from build123d import *

# Parameters (mm, degrees)
F0_R           = 4
F1_DEPTH       = 10
F3_D           = 10
F3_CSINK_D     = 12
F3_CSINK_ANGLE = 90
F4_D           = 10
F4_CSINK_D     = 12
F4_CSINK_ANGLE = 90
F6_D           = 5


with BuildPart() as f1:
    # F0 (on Front) → F1 (new body)
    with BuildSketch(Plane.XZ):
        Polygon((0, 0), (-275, 0), (-275, -150), (275, -150), (275, 0), (50, 0), align=None)
        with Locations((-49.989153, -111.041441)):
            Circle(F0_R, mode=Mode.SUBTRACT)
        with Locations((49.989153, -111.041441)):
            Circle(F0_R, mode=Mode.SUBTRACT)
        with Locations((-49.989153, -41.041441)):
            Circle(F0_R, mode=Mode.SUBTRACT)
        with Locations((49.989153, -41.041441)):
            Circle(F0_R, mode=Mode.SUBTRACT)
    extrude(amount=F1_DEPTH)

    # F3 (through all)
    with Locations(Plane.XZ.offset(10)):
        with Locations((-132.18379, -88.733308)):
            CounterSinkHole(F3_D / 2, F3_CSINK_D / 2, counter_sink_angle=F3_CSINK_ANGLE)

    # F4 (through all)
    with Locations(Plane.XZ.offset(10)):
        with Locations((-164.520353, -73.822677)):
            CounterSinkHole(F4_D / 2, F4_CSINK_D / 2, counter_sink_angle=F4_CSINK_ANGLE)

    # F6 (through all)
    with Locations(Plane.XZ.offset(10)):
        with Locations((133.962631, -73.108293)):
            Hole(F6_D / 2)


solid = f1.part
Geometry: final body of the model. Coordinates: model frame, mm. Give positions to 0.01 mm unless a question says otherwise; leave off trailing zeros. Answer as a JSON object with one key per item and string values.
1. Contact query for a flat-ended pin moving along its axis: pin 1 (8 mm diameter, centred on x = -164.52, z = -73.82, fed in from -Y). Output: stop coordinate, or through.
Ans:
{"pin 1": "passes through"}
2. Mould query, pull axis X, two halves, no side actions, for faces 1 (the cylindrical face through (-127.19, -4.44, -88.51)), 2 (the flat face through (-4, -10, -74)), 3 (the flat face through (-275, -5, -74)). Classes: pulls with the +X half, pulls with the -X half, needs draft (parallel to the pull), parting line crosses it, or undercut.
Ans:
{"face 1": "undercut", "face 2": "needs draft", "face 3": "pulls with the -X half"}
3. Ray query, probe 1 along Z at (x, y) = (-166.5, -4.5); probe 2 along Z at (x, y) = (-130, -0.75). Return the intervals inside material, ascending. Write a range as from..to.
Ans:
{"probe 1": "z = -150..-78.41, -69.23..0", "probe 2": "z = -150..-93.23, -84.24..0"}
